Work out the finished part from the listing and answer in its coordinate system (mm). Round coordinates to 2 decimals unless told otherwise and drop trailing zeros. Order: outer loops, then holes, each group sorted by start corner. A loop starts at its lowest first (then second) coordinate and runs counter-clockwise, first axis right, second up. Notation, with made-up numbers: (61, 89) - (80, 89) arc R26 ccw to (80, 113) - close; hole circle Ø4 at (6.25, 87.25). An arc over 180 degrees is marked (long way). Put each result on its own line as item: value.
```python
from build123d import *

# Parameters (mm, degrees)
F1_W     = 240
F1_H     = 240
F1_W_2   = 6
F1_H_2   = 6
F1_W_3   = 208
F1_H_3   = 208
F2_DEPTH = 3
F3_DEPTH = 25


with BuildPart() as f2:
    # F1 (on Front) → F2 (new body)
    with BuildSketch(Plane.XZ):
        with Locations((120, 120)):
            Rectangle(F1_W, F1_H)
        with Locations((6, 234)):
            Rectangle(F1_W_2, F1_H_2, mode=Mode.SUBTRACT)
        with Locations((120, 120)):
            Rectangle(F1_W_3, F1_H_3, mode=Mode.SUBTRACT)
        with Locations((6, 234)):
            Rectangle(F1_W_2, F1_H_2)
    extrude(amount=F2_DEPTH)

    # F1 (on Front) → F3 (cut)
    with BuildSketch(Plane.XZ):
        with Locations((6, 234)):
            Rectangle(F1_W_2, F1_H_2)
    extrude(amount=F3_DEPTH, mode=Mode.SUBTRACT)

    # F5: F2 across plane


with BuildPart() as f2_1:
    add(f2.part)
    add(f2.part.mirror(Plane(origin=(120, -1.5, 120), x_dir=(0, -1, 0), z_dir=(-1, 0, 0))), mode=Mode.INTERSECT)

    # F7: F2 across plane


with BuildPart() as f2_2:
    add(f2_1.part)
    add(f2_1.part.mirror(Plane(origin=(120, -1.5, 120), x_dir=(1, 0, 0), z_dir=(0, 0, 1))), mode=Mode.INTERSECT)


solid = f2_2.part
```
1) A cutting plane is placed at B-B on x = 44.5. Write down the section's boundary in (y, z).
Findings below:
outline: (-3, 0) - (0, 0) - (0, 16) - (-3, 16) - close; (-3, 224) - (0, 224) - (0, 240) - (-3, 240) - close
2) A cutting plane is placed at C-C on z = 49. Write down the section's boundary in (x, y).
Findings below:
outline: (0, -3) - (16, -3) - (16, 0) - (0, 0) - close; (224, -3) - (240, -3) - (240, 0) - (224, 0) - close
3) A cutting plane is placed at A-A on y = -1.3. Write down the section's boundary in (x, z), then the cut area to 3 significant figures.
Findings below:
outline: (0, 0) - (240, 0) - (240, 240) - (0, 240) - close; hole (3, 3) - (9, 3) - (9, 9) - (3, 9) - close; hole (3, 231) - (9, 231) - (9, 237) - (3, 237) - close; hole (16, 16) - (224, 16) - (224, 224) - (16, 224) - close; hole (231, 3) - (237, 3) - (237, 9) - (231, 9) - close; hole (231, 231) - (237, 231) - (237, 237) - (231, 237) - close
area: 14,200 mm2
4) Given pin 1 Ø1.5 at (x, y) = (6, -1) entering from -Z, flat-ended and moving along its own axis, determine where the tip first touches the part or whether it passes through.
Findings below:
pin 1: stops at z = 0
5) A straight line is drawn through the part: L1, parallel to X at y = -1.45, z = 73. Find the intervals that lie inside material, in ascending order. Write a range as from..to.
Findings below:
L1: x = 0..16, 224..240
